Can you work these out from the model? Positions are in its coordinate system, mm. Face numbers are marked on the shaded views. A direction names the side the tool comes from. Coordinates: 2 decimals unless noted, no trailing zeros. Loops run counter-clockwise (first coordinate to the right, second up) from the corner with the lowest first, then second, coordinate; pieces in that order, holes last. Notation, with made-up numbers: (75.25, 1) - (117.25, 1) arc R33 cw to (117.25, 39) - close; hole circle Ø5 at (-13, 23.25). An arc over 180 degrees is marked (long way). Put each result on its own line as item: value. Start each with the question number.
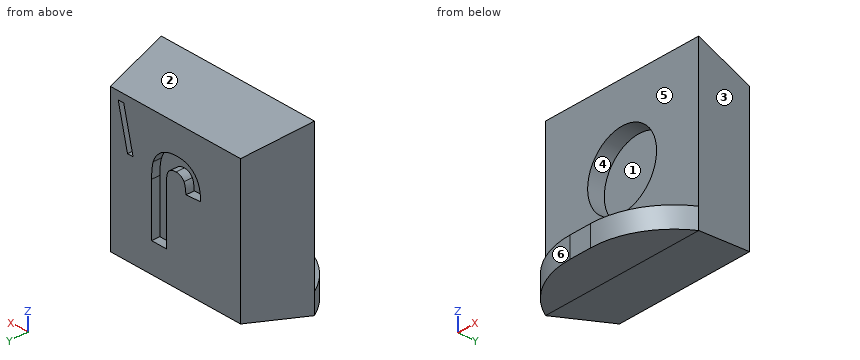
from build123d import *

# Parameters (mm, degrees)
SKETCH1_W               = 8
SKETCH1_H               = 8
BOSS_EXTRUDE1_DEPTH     = 3
CUT_EXTRUDE1_DEPTH      = 12.704699911
CUT_EXTRUDE1_DEPTH_BACK = 12.704699911
CUT_EXTRUDE2_DEPTH      = 11
SKETCH4_R               = 1.8
CUT_EXTRUDE3_DEPTH      = 0.8
SKETCH5_W               = 8
SKETCH5_H               = 1
BOSS_EXTRUDE2_DEPTH     = 2
FILLET1_R               = 4
CUT_EXTRUDE4_DEPTH      = 0.4
CUT_EXTRUDE5_DEPTH      = 0.4


with BuildPart() as part:
    # Sketch1 → Boss-Extrude1 (new body)
    with BuildSketch(Plane(origin=(0, 0, 0), x_dir=(1, 0, 0), z_dir=(0, 1, 0))):
        with Locations((4, 4)):
            Rectangle(SKETCH1_W, SKETCH1_H)
    extrude(amount=BOSS_EXTRUDE1_DEPTH)

    # Sketch2 → Cut-Extrude1 (cut, two sides: drawn at the far end of the back side and taken through both)
    with BuildSketch(Plane.XY.offset(-CUT_EXTRUDE1_DEPTH_BACK)):
        Polygon((0, 0), (0.6, 3), (0, 3), align=None)
        Polygon((8, 0), (7.4, 3), (8, 3), align=None)
    extrude(amount=CUT_EXTRUDE1_DEPTH + CUT_EXTRUDE1_DEPTH_BACK, mode=Mode.SUBTRACT)

    # Sketch3 → Cut-Extrude2 (cut)
    with BuildSketch(Plane(origin=(0, 0, 0), x_dir=(0, 0, -1), z_dir=(1, 0, 0))):
        Polygon((0, 0), (0.6, 3), (0, 3), align=None)
        Polygon((8, 3), (7.4, 3), (8, 0), align=None)
    extrude(amount=CUT_EXTRUDE2_DEPTH, mode=Mode.SUBTRACT)

    # Sketch4 → Cut-Extrude3 (cut)
    with BuildSketch(Plane.XZ):
        with Locations(Location((4, -3.75, 0), (0, 0, 270))):
            Circle(SKETCH4_R)
    extrude(amount=-CUT_EXTRUDE3_DEPTH, mode=Mode.SUBTRACT)

    # Sketch5 → Boss-Extrude2 (add)
    with BuildSketch(Plane.XZ):
        with Locations((4, -7.5)):
            Rectangle(SKETCH5_W, SKETCH5_H)
    extrude(amount=BOSS_EXTRUDE2_DEPTH)

    # Fillet1
    # the kernel refuses this fillet: 4 mm, written as the material it takes off along each edge
    with BuildSketch(Plane(origin=(8, -2, -16.660254038), x_dir=(0, 1, 0), z_dir=(0, 0, 1)), Plane(origin=(0, -2, 1.660254038), x_dir=(0, 1, 0), z_dir=(0, 0, -1))) as fillet1_piece_1:
        with BuildLine():
            CenterArc((4, 3.464101615), FILLET1_R, 180, 60)
            Line((0, 3.464101615), (-0.08, 3.464101615))
            Line((-0.08, 3.464101615), (-0.08, 0))
            Line((-0.08, 0), (0, -0.08))
            ThreePointArc((0, -0.08), (1, -0.08), (1.96, -0.069282032))
            Line((1.96, -0.069282032), (2, 0))
        make_face()
    extrude(amount=18.320508076, mode=Mode.SUBTRACT)

    # Sketch6 → Cut-Extrude4 (cut)
    with BuildSketch(Plane(origin=(0, 3, 0), x_dir=(1, 0, 0), z_dir=(0, 1, 0))):
        with BuildLine():
            Line((4.478635236, 6.002856352), (5.247866005, 6.002856352))
            Line((5.247866005, 6.002856352), (5.247866005, 3.481221736))
            add(Edge.make_bspline(
                [(5.247866005, 3.481221736), (5.247522255, 3.441153869), (5.246855206, 3.363401883), (5.242756502, 3.250390465), (5.236658321, 3.14454193), (5.227277222, 3.045871471), (5.21405872, 2.954592388), (5.200049867, 2.869976575), (5.183041427, 2.792451692), (5.167800036, 2.743951306), (5.160526262, 2.72080507)],
                knots=[0, 0, 0, 0, 1.251619961, 2.428777588, 3.532126049, 4.56323557, 5.523704531, 6.412540087, 7.242403515, 8, 8, 8, 8], degree=3))
            add(Edge.make_bspline(
                [(5.160526262, 2.72080507), (5.150361081, 2.692282601), (5.130243602, 2.635834988), (5.091141653, 2.555314881), (5.046176431, 2.479084315), (4.995474484, 2.406812938), (4.939514717, 2.338210987), (4.876399077, 2.275086649), (4.8083478, 2.215238098), (4.733446681, 2.161145289), (4.653580791, 2.110709794), (4.566475051, 2.068688963), (4.473843299, 2.032340387), (4.374908104, 2.002816628), (4.269640778, 1.979716073), (4.158311001, 1.962901894), (4.040770466, 1.95334773), (3.960490164, 1.952175274), (3.919340364, 1.9515743)],
                knots=[0, 0, 0, 0, 0.925533072, 1.831683394, 2.73255258, 3.630007683, 4.529542467, 5.436465751, 6.357118906, 7.298274949, 8.259461937, 9.242242071, 10.251058183, 11.300341426, 12.396409345, 13.544807631, 14.74152597, 16, 16, 16, 16], degree=3))
            add(Edge.make_bspline(
                [(3.919340364, 1.9515743), (3.871225528, 1.952737211), (3.777685944, 1.954998015), (3.641661475, 1.97000769), (3.514100564, 1.996260242), (3.395387048, 2.034179675), (3.284307874, 2.08131717), (3.182206561, 2.140114726), (3.088540477, 2.209392701), (3.003918711, 2.289363431), (2.928299433, 2.379218215), (2.863026475, 2.479745415), (2.80762712, 2.589893743), (2.762984692, 2.710161506), (2.727739397, 2.839972913), (2.702317462, 2.979601288), (2.687147894, 3.129126134), (2.684913172, 3.2319872), (2.683763441, 3.284907634)],
                knots=[0, 0, 0, 0, 1.114068574, 2.165849827, 3.164101702, 4.124467949, 5.046988974, 5.952942428, 6.846011651, 7.738523925, 8.642829306, 9.558838605, 10.50752403, 11.491963144, 12.524197802, 13.618364352, 14.774685164, 16, 16, 16, 16], degree=3))
            Line((2.683763441, 3.284907634), (3.45299421, 3.336189685))
            add(Edge.make_bspline(
                [(3.45299421, 3.336189685), (3.454375767, 3.307862598), (3.45702498, 3.25354382), (3.464380935, 3.175240866), (3.473682687, 3.103271277), (3.485853837, 3.037851064), (3.498960823, 2.978427444), (3.515987002, 2.926169857), (3.533886556, 2.879240769), (3.549608387, 2.851783511), (3.557160877, 2.838593531)],
                knots=[0, 0, 0, 0, 1.326609226, 2.543847584, 3.678365909, 4.719972403, 5.656527627, 6.521948534, 7.28997025, 8, 8, 8, 8], degree=3))
            add(Edge.make_bspline(
                [(3.557160877, 2.838593531), (3.56872297, 2.821148121), (3.59147861, 2.786813382), (3.632990929, 2.742071605), (3.677558537, 2.702955843), (3.727619554, 2.672203009), (3.781780527, 2.648016829), (3.840448037, 2.63044225), (3.903460331, 2.619785853), (3.946808463, 2.61876437), (3.969019851, 2.618240967)],
                knots=[0, 0, 0, 0, 1.023658308, 2.014687051, 2.979722519, 3.920049697, 4.880550909, 5.878122304, 6.912759386, 8, 8, 8, 8], degree=3))
            add(Edge.make_bspline(
                [(3.969019851, 2.618240967), (3.991477248, 2.618659453), (4.034647527, 2.619463917), (4.09686091, 2.626779219), (4.154063033, 2.638632824), (4.206285054, 2.655294856), (4.253703868, 2.676924623), (4.295268393, 2.704596166), (4.33276969, 2.735732915), (4.36516489, 2.773188264), (4.392766236, 2.818318957), (4.415812105, 2.873248962), (4.43563784, 2.938204221), (4.450960178, 3.01367855), (4.464002509, 3.098949399), (4.472183692, 3.194770716), (4.478064386, 3.300859295), (4.478439634, 3.37517575), (4.478635236, 3.413914044)],
                knots=[0, 0, 0, 0, 0.980314827, 1.884477813, 2.730827652, 3.527503874, 4.27366112, 4.998269146, 5.70163477, 6.396145331, 7.150281155, 8.001758491, 8.990432449, 10.111292654, 11.361572691, 12.75538406, 14.308707205, 16, 16, 16, 16], degree=3))
            Line((4.478635236, 3.413914044), (4.478635236, 6.002856352))
        make_face()
    extrude(amount=-CUT_EXTRUDE4_DEPTH, mode=Mode.SUBTRACT)

    # Sketch7 → Cut-Extrude5 (cut)
    with BuildSketch(Plane(origin=(0, 3, 0), x_dir=(1, 0, 0), z_dir=(0, 1, 0))):
        Polygon((6.21271865, 2.977310221), (6.502782752, 2.977310221), (6.989962239, 0.977310221), (6.700298778, 0.977310221), align=None)
    extrude(amount=-CUT_EXTRUDE5_DEPTH, mode=Mode.SUBTRACT)


solid = part.part
Q1. I want a section at C-C on y = -0.3. List the corners of the cut face in (x, z) for me, and give its area (3 significant figures).
Q2. I want a section at A-A on z = -3.75. List the corners of the cut face in (x, y) for me.
Q3. Will these pins go through, and if not, where does the flat tip stop? pin 1 (3 mm diameter, centred on x = 3, z = -1, fed in from -Y); pin 2 (1.5 mm diameter, centred on y = 1.5, z = -3.5, fed in from -X); pin 3 (0.6 mm diameter, centred on x = 3, y = -1.5, fed in from +Z).
Q4. On a 3-axis mill with a long thin cutter (end or side, diameter ignored), from which of +Z, -Z, +X, -X, +Y, -Y can I reach the whole of each face in a straight line? I mean the marked faces 4, 5 and 6. Say none if no direction works.
Q5. Please list where these lines run through material, in increasing order: line 1 along Y through (x, z) = (3, -4.5); line 2 along Y through (x, z) = (6, -2.5); line 3 along X through (y, z) = (0.55, -3.75). Write a range as [from, to].
Q6. I want a section at D-D on z = -0.75. List the corners of the cut face in (x, y) for me.
Q7. I want a section at B-B on x = 2.5. List the corners of the cut face in (y, z) for me, and give its area (3 significant figures).
Q8. We'd pull the mould along Z, two halves only. Please class the marked faces 1, 2 and 3: released by +Z, released by -Z, zero draft, split by the parting line, or undercut.
Calculated:
1. outline: (0.19, -8) - (7.81, -8) - (7.81, -7) - (0.19, -7) - close
1. area: 7.62 mm2
2. outline: (0, 0) - (2.2, 0) - (2.2, 0.8) - (5.8, 0.8) - (5.8, 0) - (8, 0) - (7.4, 3) - (5.25, 3) - (5.25, 2.6) - (4.48, 2.6) - (4.48, 3) - (0.6, 3) - close
3. pin 1: y = 0
3. pin 2: x = 0.15
3. pin 3: z = -7
4. face 4: -Y
4. face 5: +Z, +X, -X, -Y
4. face 6: +Z, -Z, -X, -Y
5. line 1: [0.8, 3]
5. line 2: [0, 3]
5. line 3: [0.11, 2.2], [5.8, 7.89]
6. outline: (0, 0) - (8, 0) - (7.4, 3) - (0.6, 3) - close
7. outline: (-1.88, -8) - (0, -8) - (3, -7.4) - (3, -0.6) - (0, 0) - (0, -2.76) - (0.8, -2.76) - (0.8, -4.74) - (0, -4.74) - (0, -7) - (-1.88, -7) - close
7. area: 22.5 mm2
8. face 1: undercut
8. face 2: released by +Z
8. face 3: zero draft
